from build123d import *

# Parameters (mm, degrees)
F0_R          = 10
F1_DEPTH      = 15
F3_START      = -10
F2_R          = 10
F3_DEPTH      = 20
F5_DEPTH      = 10
F5_DEPTH_BACK = 10
F6_W          = 10
F6_H          = 10
F7_DEPTH      = 110.001


with BuildPart() as f1:
    # F0 (on Top) → F1 (new body)
    with BuildSketch(Plane.XY):
        with BuildLine():
            Line((55, 75), (-55, 75))
            Line((-55, 75), (-55, 6))
            ThreePointArc((-55, 6), (-53.2426406871, 1.7573593129), (-49, 0))
            Line((-49, 0), (49, 0))
            ThreePointArc((49, 0), (53.2426406871, 1.7573593129), (55, 6))
            Line((55, 6), (55, 75))
        make_face()
        with Locations((-25, 20)):
            Circle(F0_R, mode=Mode.SUBTRACT)
        with BuildLine():
            ThreePointArc((15, 20), (25, 30), (35, 20))
            ThreePointArc((35, 20), (25, 10), (15, 20))
        make_face(mode=Mode.SUBTRACT)
    extrude(amount=F1_DEPTH)

    # F2 (on face) → F3 (join)
    with BuildSketch(Plane(origin=(0, 75, 0), x_dir=(-1, 0, 0), z_dir=(0, 1, 0)).offset(F3_START)):
        with BuildLine():
            ThreePointArc((50, 15), (32.3223304703, 22.3223304703), (25, 40))
            Line((25, 40), (25, 95))
            ThreePointArc((25, 95), (0, 120), (-25, 95))
            Line((-25, 95), (-25, 40))
            ThreePointArc((-25, 40), (-32.3223304703, 22.3223304703), (-50, 15))
            Line((-50, 15), (50, 15))
        make_face()
        with Locations((0, 95)):
            Circle(F2_R, mode=Mode.SUBTRACT)
    extrude(amount=-F3_DEPTH)

    # F4 (on Right) → F5 (join, two sides)
    with BuildSketch(Plane.YZ) as f5_sk:
        Polygon((45, 75), (0, 15), (45, 15), align=None)
    extrude(amount=F5_DEPTH)
    extrude(f5_sk.sketch, amount=-F5_DEPTH_BACK)

    # F6 (on face) → F7 (cut, through all)
    with BuildSketch(Plane.YZ.offset(55)):
        with Locations((70, 10)):
            Rectangle(F6_W, F6_H)
    extrude(amount=-F7_DEPTH, mode=Mode.SUBTRACT)


solid = f1.part
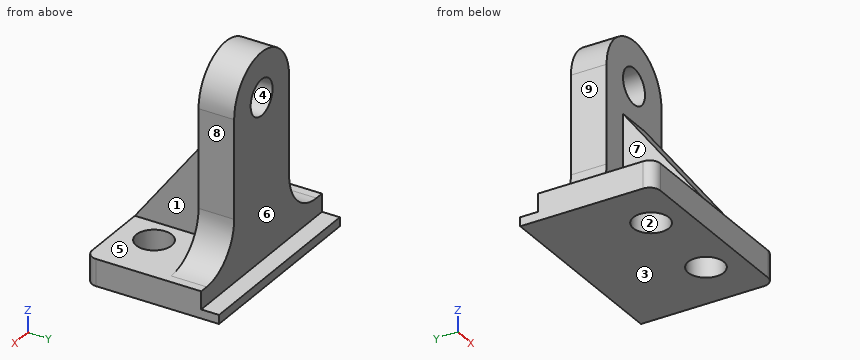
Design review of the part built by this model. Coordinates are the model's own, in mm. Face numbers are marked on the shaded views. A direction names the side the tool comes from. Give positions to 0.01 mm unless a question says otherwise; leave off trailing zeros. Write each loop counter-clockwise with the first axis right and the second up, starting at its lowest first coordinate (ties: lowest second). Pieces come first, ordered by that corner, then holes. Notation, with made-up numbers: M -1.5,-25.75 L 29.5,-25.75 A17 ccw 29.5,-21.75 Z; hole C -10.5,-36.75 d5. An arc over 180 degrees is marked long. Answer as a JSON object with one key per item and string values. Group by question number.
1) We need section B-B (y = 55). Give the boundary of the cut face in (x, z).
2) Mouldability with a two-part tool opening along X and no side actions: class the marked faces 1, 2, 3 and 4 as released by +X, released by -X, zero draft, split by the parting line, or undercut.
3) We need section D-D (x = 41.5). Give the boundary of the cut face in (y, z).
4) We need section A-A (z = 10). Give the boundary of the cut face in (x, y).
5) Clearance check with flat-ended pins moving along their axes: pin 1 Ø4 at (x, y) = (-7.5, 35) entering from +Z; pin 2 Ø4 at (x, y) = (22.5, 31) entering from -Z; pin 3 Ø13.5 at (x, y) = (27.5, 45) entering from +Z; pin 4 Ø10 at (y, z) = (66.5, 62.5) entering from -X. State where each tip first meets the part, or that it passes through.
6) We need section C-C (x = -7). Give the boundary of the cut face in (y, z).
7) For line 1 along Y through (x, z) = (-25, 6); line 2 along X through (y, z) = (34.5, 44); line 3 along Z through (x, y) = (0, 51), list the stretches that pass through material, from the lowest coordinate up.
8) Tool access review of the marked faces 5, 6, 7, 8 and 9: name each direction out of +Z, -Z, +X, -X, +Y, -Y from which nothing blocks a thin tool from reaching the whole face with its end or side.
Answer key:
{
 "1": {"outline": "M -55,0 L 55,0 L 55,15 L 50,15 A25 cw 25,40 L 25,95 A25 ccw -25,95 L -25,40 A25 cw -50,15 L -55,15 Z; hole C 0,95 d20"},
 "2": {"face 1": "released by +X", "face 2": "undercut", "face 3": "zero draft", "face 4": "undercut"},
 "3": {"outline": "M 0,0 L 75,0 L 75,5 L 65,5 L 65,16.49 L 45,16.49 L 45,15 L 0,15 Z"},
 "4": {"outline": "M -55,6 A6 ccw -49,0 L 49,0 A6 ccw 55,6 L 55,65 L -55,65 Z; hole C -25,20 d20; hole C 25,20 d20"},
 "5": {"pin 1": "stops at z = 64.33", "pin 2": "stops at z = 0", "pin 3": "stops at z = 108.94", "pin 4": "stops at x = -25"},
 "6": {"outline": "M 0,0 L 75,0 L 75,5 L 65,5 L 65,87.86 L 45,87.86 L 45,75 L 0,15 Z; M 45,102.14 L 65,102.14 L 65,119 L 45,119 Z"},
 "7": {"line 1": "y = 0 to 10, 30 to 65", "line 2": "x = -10 to 10", "line 3": "z = 0 to 85, 105 to 120"},
 "8": {"face 5": "+Z, +X, -Y", "face 6": "+Z, +X, -X, +Y", "face 7": "+Z, -X, -Y", "face 8": "+Z, +X, +Y, -Y", "face 9": "+Z, -X, +Y, -Y"}
}
